The listing builds one solid part. Answer for the finished solid, in the listing's coordinates (mm). Give positions to 0.01 mm unless a question says otherwise; leave off trailing zeros. Order: outer loops, then holes, each group sorted by start corner. A loop starts at its lowest first (then second) coordinate and runs counter-clockwise, first axis right, second up. Notation, with made-up numbers: (26.25, -10) - (54.25, -10) arc R22 ccw to (54.25, 3) - close; hole circle Ø3 at (41, 31.25). An arc over 180 degrees is marked (long way). Answer in a Markdown table with one row per item.
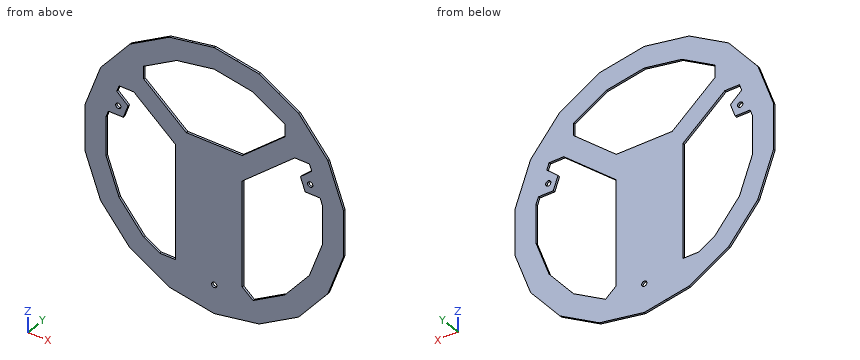
from build123d import *

# Parameters (mm, degrees)
BOSS_EXTRUDE1_DEPTH    = 1.2
BOSS_EXTRUDE17_DEPTH   = 1.2
BOSS_EXTRUDE17_2_DEPTH = 1.2
BOSS_EXTRUDE17_3_DEPTH = 1.2
SKETCH18_W             = 18
SKETCH18_H             = 25
BOSS_EXTRUDE18_DEPTH   = 1.2
BOSS_EXTRUDE19_DEPTH   = 1.2
BOSS_EXTRUDE20_DEPTH   = 1.2
BOSS_EXTRUDE22_DEPTH   = 1.2
BOSS_EXTRUDE26_DEPTH   = 1.2
BOSS_EXTRUDE28_DEPTH   = 1.2
BOSS_EXTRUDE23_DEPTH   = 1.2
SKETCH38_R             = 1.5
CUT_EXTRUDE2_DEPTH     = 1.2
BOSS_EXTRUDE29_DEPTH   = 1.2
SKETCH37_R             = 1.5
CUT_EXTRUDE3_DEPTH     = 1.2
BOSS_EXTRUDE30_DEPTH   = 1.2
CUT_EXTRUDE4_DEPTH     = 1.2


with BuildPart() as part:
    # Sketch1 → Boss-Extrude1 (new body)
    with BuildSketch(Plane(origin=(0, 0, 0), x_dir=(1, 0, 0), z_dir=(0, 1, 0))):
        Polygon((0, 75), (-25.651510749, 70.476946559), (-48.209070726, 57.453333234), (-64.951905284, 37.5), (-73.860581476, 13.023613325), (-73.860581476, -13.023613325), (-64.951905284, -37.5), (-48.209070726, -57.453333234), (-25.651510749, -70.476946559), (0, -75), (25.651510749, -70.476946559), (48.209070726, -57.453333234), (64.951905284, -37.5), (73.860581476, -13.023613325), (73.860581476, 13.023613325), (64.951905284, 37.5), (48.209070726, 57.453333234), (25.651510749, 70.476946559), align=None)
        Polygon((0, 62.814880657), (-21.483954485, 59.026679829), (-40.37662699, 48.118990273), (-54.399282385, 31.407440329), (-61.860581476, 10.907689557), (-61.860581476, -10.907689557), (-54.399282385, -31.407440329), (-40.37662699, -48.118990273), (-21.483954485, -59.026679829), (0, -62.814880657), (21.483954485, -59.026679829), (40.37662699, -48.118990273), (54.399282385, -31.407440329), (61.860581476, -10.907689557), (61.860581476, 10.907689557), (54.399282385, 31.407440329), (40.37662699, 48.118990273), (21.483954485, 59.026679829), align=None, mode=Mode.SUBTRACT)
    extrude(amount=BOSS_EXTRUDE1_DEPTH)



with BuildPart() as body_2:
    # Sketch15 → Boss-Extrude17 (new body)
    with BuildSketch(Plane.XZ):
        Polygon((0, -101.401091909), (34.681215988, -95.285857807), (36.930290738, -93.987353894), (36.930290738, -84.749749587), (31.902845145, -87.652346653), (0, -93.277679014), (-31.902845145, -87.652346653), (-36.930290738, -84.749749587), (-36.930290738, -93.987353894), (-34.681215988, -95.285857807), align=None)
    extrude(amount=-BOSS_EXTRUDE17_DEPTH)


with BuildPart() as body_3:
    # Sketch15 → Boss-Extrude17 2 (new body)
    with BuildSketch(Plane.XZ):
        Polygon((92.620527368, -37.5), (99.860581476, -17.608114823), (99.860581476, 17.608114823), (92.620527368, 37.5), (84.107105188, 37.5), (91.860581476, 16.197498978), (91.860581476, -16.197498978), (84.107105188, -37.5), align=None)
    extrude(amount=-BOSS_EXTRUDE17_2_DEPTH)


with BuildPart() as body_4:
    # Sketch15 → Boss-Extrude17 3 (new body)
    with BuildSketch(Plane.XZ):
        Polygon((-92.620527368, 37.5), (-99.860581476, 17.608114823), (-99.860581476, -17.608114823), (-92.620527368, -37.5), (-84.107105188, -37.5), (-91.860581476, -16.197498978), (-91.860581476, 16.197498978), (-84.107105188, 37.5), align=None)
    extrude(amount=-BOSS_EXTRUDE17_3_DEPTH)


with BuildPart() as part_1:
    add(part.part)

    add(body_2.part)  # Boss-Extrude18 merges body 2

    add(body_3.part)  # Boss-Extrude18 merges body 3

    add(body_4.part)  # Boss-Extrude18 merges body 4
    # Sketch18 → Boss-Extrude18 (add)
    with BuildSketch(Plane.XZ):
        with Locations((-82.860581476, 0)):
            Rectangle(SKETCH18_W, SKETCH18_H)
        with Locations((82.860581476, 0)):
            Rectangle(SKETCH18_W, SKETCH18_H)
        Polygon((-12.5, -72.795912741), (-12.5, -91.073591755), (0, -93.277679014), (12.5, -91.073591755), (12.5, -72.795912741), (0, -75), align=None)
    extrude(amount=-BOSS_EXTRUDE18_DEPTH)

    # Sketch19 → Boss-Extrude19 (add)
    with BuildSketch(Plane.XZ):
        Polygon((-91.860581476, 16.197498978), (-82.860581476, 12.5), (-91.860581476, 12.5), align=None)
        Polygon((-91.860581476, -16.197498978), (-82.860581476, -12.5), (-91.860581476, -12.5), align=None)
        Polygon((91.860581476, 16.197498978), (82.860581476, 12.5), (91.860581476, 12.5), align=None)
        Polygon((91.860581476, -16.197498978), (82.860581476, -12.5), (91.860581476, -12.5), align=None)
        Polygon((22.201422573, -89.362969204), (12.5, -81.934752248), (12.5, -91.073591755), align=None)
        Polygon((-12.5, -81.934752248), (-12.5, -91.073591755), (-22.201422573, -89.362969204), align=None)
    extrude(amount=-BOSS_EXTRUDE19_DEPTH)

    # Sketch20 → Boss-Extrude20 (add)
    with BuildSketch(Plane.XZ):
        Polygon((-36.930290738, 63.965139896), (-36.930290738, 91.965139896), (-32.052421992, 91.965139896), (-12.825755375, 72.738473279), (-25.651510749, 70.476946559), align=None)
        Polygon((36.930290738, 63.965139896), (36.930290738, 91.965139896), (32.052421992, 91.965139896), (12.825755375, 72.738473279), (25.651510749, 70.476946559), align=None)
    extrude(amount=-BOSS_EXTRUDE20_DEPTH)

    # Sketch24 → Boss-Extrude22 (add)
    with BuildSketch(Plane(origin=(0, 1.2, 0), x_dir=(1, 0, 0), z_dir=(0, 1, 0))):
        Polygon((-36.930290738, 93.987353894), (-36.930290738, 80.130947434), (-30.513659724, 83.835591077), (-17.889679207, 86.061539446), (17.889679207, 86.061539446), (30.513659724, 83.835591077), (36.930290738, 80.130947434), (36.930290738, 93.987353894), (34.681215988, 95.285857807), (0, 101.401091909), (-34.681215988, 95.285857807), align=None)
    extrude(amount=-BOSS_EXTRUDE22_DEPTH)

    # Sketch27 → Boss-Extrude26 (add)
    with BuildSketch(Plane.XZ):
        Polygon((-50.923286541, 35.549970864), (-43.852622834, 43.976459738), (-16, 20.60533419), (16, 20.60533419), (43.852622834, 43.976459738), (50.923286541, 35.549970864), (16, 6.245854008), (16, -59.993648966), (0, -62.814880657), (-16, -59.993648966), (-16, 6.245854008), align=None)
    extrude(amount=-BOSS_EXTRUDE26_DEPTH)

    # Sketch43 → Boss-Extrude28 (add)
    with BuildSketch(Plane.XZ):
        Polygon((-40.37662699, 48.118990273), (-40.37662699, 41.059752907), (-43.852622834, 43.976459738), align=None)
        Polygon((40.37662699, 48.118990273), (40.37662699, 41.059752907), (43.852622834, 43.976459738), align=None)
        Polygon((54.399282385, 31.407440329), (45.986410894, 31.407440329), (50.923286541, 35.549970864), align=None)
        Polygon((-54.399282385, 31.407440329), (-45.986410894, 31.407440329), (-50.923286541, 35.549970864), align=None)
        Polygon((-22.128355545, -58.654634704), (-16, -53.512333827), (-16, -59.993648966), (-21.483954485, -59.026679829), align=None)
        Polygon((16, -59.993648966), (16, -53.512333827), (22.128355545, -58.654634704), (21.483954485, -59.026679829), align=None)
    extrude(amount=-BOSS_EXTRUDE28_DEPTH)

    # Sketch26 → Boss-Extrude23 (add)
    with BuildSketch(Plane(origin=(0, 1.2, 0), x_dir=(1, 0, 0), z_dir=(0, 1, 0))):
        Polygon((-36.930290738, 93.987353894), (-45.930290738, 88.791201472), (-45.930290738, 74.934795011), (-36.930290738, 80.130947434), align=None)
        Polygon((36.930290738, 93.987353894), (45.930290738, 88.791201472), (45.930290738, 74.934795011), (36.930290738, 80.130947434), align=None)
    extrude(amount=-BOSS_EXTRUDE23_DEPTH)

    # Sketch38 → Cut-Extrude2 (cut)
    with BuildSketch(Plane(origin=(0, 1.2, 0), x_dir=(1, 0, 0), z_dir=(0, 1, 0))):
        with Locations(Location((0, 58.81204127, 0), (0, 0, 270))):
            Circle(SKETCH38_R)
    extrude(amount=-CUT_EXTRUDE2_DEPTH, mode=Mode.SUBTRACT)

    # Sketch34 → Boss-Extrude29 (add)
    with BuildSketch(Plane(origin=(0, 1.2, 0), x_dir=(1, 0, 0), z_dir=(0, 1, 0))):
        Polygon((-60.493893717, -14.662633313), (-55.705611711, -27.818330004), (-49.244310391, -22.180174279), (-50.612390964, -18.421403796), (-51.980471537, -14.662633313), align=None)
        Polygon((50.612390964, -18.421403796), (49.244310391, -22.180174279), (55.705611711, -27.818330004), (60.493893717, -14.662633313), (51.980471537, -14.662633313), align=None)
    extrude(amount=-BOSS_EXTRUDE29_DEPTH)

    # Sketch37 → Cut-Extrude3 (cut)
    with BuildSketch(Plane(origin=(0, 1.2, 0), x_dir=(1, 0, 0), z_dir=(0, 1, 0))):
        with Locations(Location((-54.84814578, -19.96309247, 0), (0, 0, 270))):
            Circle(SKETCH37_R)
        with Locations(Location((54.84814578, -19.96309247, 0), (0, 0, 270))):
            Circle(SKETCH37_R)
    extrude(amount=-CUT_EXTRUDE3_DEPTH, mode=Mode.SUBTRACT)

    # Sketch44 → Boss-Extrude30 (add)
    with BuildSketch(Plane.XZ):
        Polygon((-22.128355545, 11.388154885), (-16, 6.245854008), (-16, -53.512333827), (-22.128355545, -58.654634704), (-31.035081933, -53.512333827), (-22.128355545, -53.512333827), align=None)
    extrude(amount=-BOSS_EXTRUDE30_DEPTH)

    # Sketch46 → Cut-Extrude4 (cut)
    with BuildSketch(Plane.XZ):
        Polygon((-73.860581476, -13.023613325), (-84.107105188, -37.5), (-92.620527368, -37.5), (-99.860581476, -17.608114823), (-99.860581476, 17.608114823), (-92.620527368, 37.5), (-84.107105188, 37.5), (-73.860581476, 12.5), align=None)
        Polygon((73.860581476, 12.5), (84.107105188, 37.5), (92.620527368, 37.5), (99.860581476, 17.608114823), (99.860581476, -17.608114823), (92.620527368, -37.5), (84.107105188, -37.5), (73.860581476, -12.5), align=None)
        Polygon((-12.5, -72.795912741), (-45.930290738, -74.934795011), (-45.930290738, -88.791201472), (-34.681215988, -95.285857807), (0, -101.401091909), (34.681215988, -95.285857807), (45.930290738, -88.791201472), (45.930290738, -74.934795011), (12.5, -72.795912741), (0, -75), align=None)
        Polygon((-36.930290738, 63.965139896), (-36.930290738, 91.965139896), (-32.052421992, 91.965139896), (-12.825755375, 72.738473279), (-25.651510749, 70.476946559), align=None)
        Polygon((12.825755375, 72.738473279), (32.052421992, 91.965139896), (36.930290738, 91.965139896), (36.930290738, 63.965139896), (25.651510749, 70.476946559), align=None)
    extrude(amount=-CUT_EXTRUDE4_DEPTH, mode=Mode.SUBTRACT)


solid = part_1.part
Item 1: Find section D-D on y = 1. Count the separate pieces of the cut face and the enclosed holes in it, then the cut area to 3 significant figures.
Answer block:
| item | result |
|---|---|
| separate pieces | 1 |
| enclosed holes | 6 |
| area | 9,370 mm² |
Item 2: Find section A-A on z = -22.5. Write down the section's boundary in (x, y).
Answer block:
| item | result |
|---|---|
| outline | (-70.41, 0) - (-57.64, 0) - (-57.64, 1.2) - (-70.41, 1.2) - close; (-22.13, 0) - (16, 0) - (16, 1.2) - (-22.13, 1.2) - close; (57.64, 0) - (70.41, 0) - (70.41, 1.2) - (57.64, 1.2) - close |
Item 3: Find section B-B on x = -8. Write down the section's boundary in (y, z), then the cut area to 3 significant figures.
Answer block:
| item | result |
|---|---|
| outline | (0, -73.59) - (1.2, -73.59) - (1.2, 20.61) - (0, 20.61) - close; (0, 61.4) - (1.2, 61.4) - (1.2, 73.59) - (0, 73.59) - close |
| area | 128 mm² |
Item 4: Consider line 1 (X direction, y = 0.9, z = 6); line 2 (X direction, y = 1, z = -20); line 3 (Z direction, x = 19.5, y = 0.9). Determine where each line is inside the solid, lowest interval first.
Answer block:
| item | result |
|---|---|
| line 1 | -73.86 to -61.86, -22.13 to 16, 61.86 to 73.86 |
| line 2 | -71.32 to -58.55, -22.13 to 16, 58.55 to 71.32 |
| line 3 | -71.56 to -56.45, 9.18 to 23.54, 59.38 to 71.56 |
Item 5: Each of these flat-tipped pins is pushed along its axis until it touches: P1, Ø2.5, axis at x = -54.85, z = 19.96, coming from the +Y side; P2, Ø0.6, axis at y = 1, z = 45, coming from the +X side. Where does it stop, or does it pass through?
Answer block:
| item | result |
|---|---|
| P1 | through |
| P2 | x = 58.91 |
Item 6: Find section C-C on z = 51.5. Write down the section's boundary in (x, y), then the cut area to 3 significant figures.
Answer block:
| item | result |
|---|---|
| outline | (-53.2, 0) - (-34.52, 0) - (-34.52, 1.2) - (-53.2, 1.2) - close; (34.52, 0) - (53.2, 0) - (53.2, 1.2) - (34.52, 1.2) - close |
| area | 44.8 mm² |
